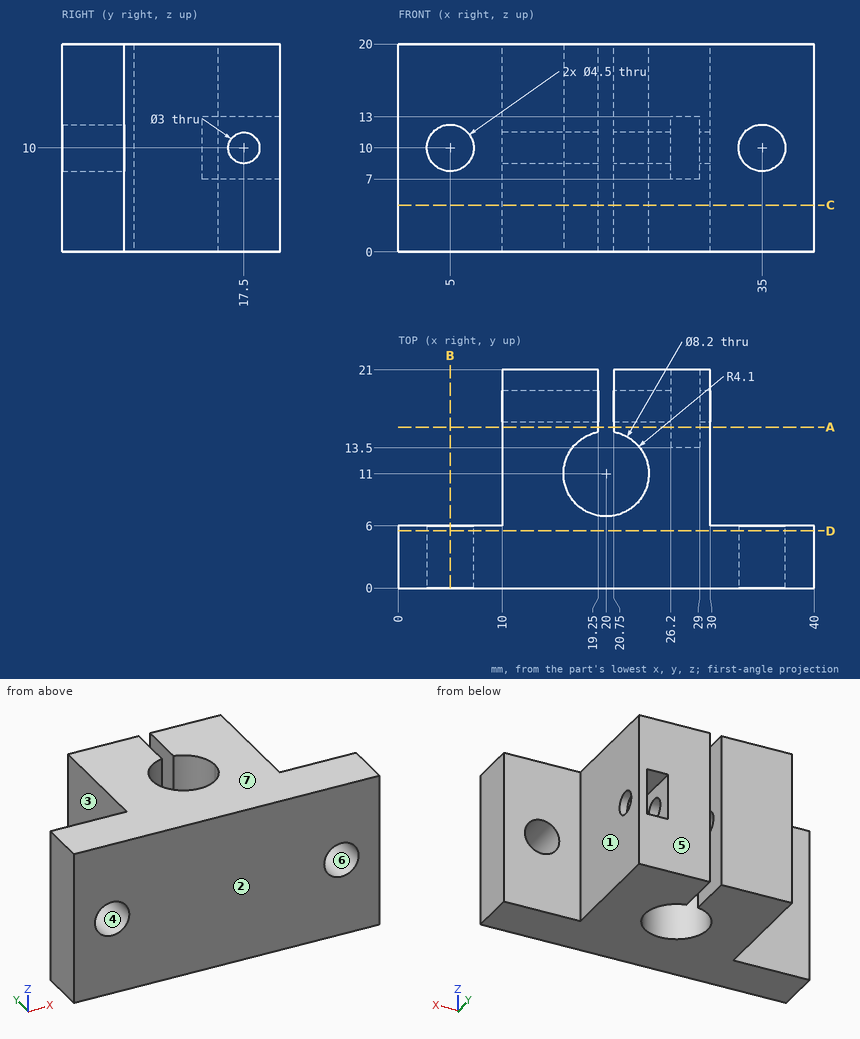
Can you work these out from the drawing? Everything is in mm from the part's minimum corner. A direction names the side the tool comes from. Round coordinates to 2 decimals unless told otherwise and drop trailing zeros. Write each loop counter-clockwise with the first axis right and the second up, starting at its lowest first coordinate (ties: lowest second). Pieces come first, ordered by that corner, then holes. Notation, with made-up numbers: (73.5, 60) - (129.5, 60) arc R20 ccw to (129.5, 93) - close; hole circle Ø6 at (8, 71). An arc over 180 degrees is marked (long way). Use a Markdown table: item, result.
Q1. Please list where these lines run through material, in increasing order: L1, parallel to X at y = 18, z = 12.25; L2, parallel to X at y = 16.5, z = 15; L3, parallel to Z at x = 35, y = 1.25.
Output values:
| item | result |
|---|---|
| L1 | 10 to 19.25, 20.75 to 26.2, 29 to 30 |
| L2 | 10 to 19.25, 20.75 to 30 |
| L3 | 0 to 7.75, 12.25 to 20 |
Q2. For pin 1 (7.5 mm diameter, centred on y = 10.5, z = 9.5, fed in from -X); pin 2 (7 mm diameter, centred on x = 35, z = 10, fed in from +Y); pin 3 (6 mm diameter, centred on x = 35.5, y = 14.5, fed in from -Z); pin 4 (5 mm diameter, centred on y = 16, z = 9.5, fed in from +X), each with a flat end and sliding along its axis, tell me the tip position at first contact or that it passes through.
Output values:
| item | result |
|---|---|
| pin 1 | x = 10 |
| pin 2 | y = 6 |
| pin 3 | through |
| pin 4 | x = 30 |
Q3. Thinking about a two-plate mould opening in Z: for the marked faces 4, 5, 6 and 7, which applies, released by +Z, released by -Z, zero draft, split by the parting line, or undercut?
Output values:
| item | result |
|---|---|
| face 4 | undercut |
| face 5 | zero draft |
| face 6 | undercut |
| face 7 | released by +Z |
Q4. I want a section at A-A (y = 15.5). List the corners of the cut face in (x, z) for me.
Output values:
| item | result |
|---|---|
| outline | (10, 0) - (19.25, 0) - (19.25, 20) - (10, 20) - close; (20.75, 0) - (30, 0) - (30, 20) - (20.75, 20) - close; hole (26.2, 7) - (29, 7) - (29, 13) - (26.2, 13) - close |
Q5. I want a section at C-C (z = 4.5). List the corners of the cut face in (x, y) for me.
Output values:
| item | result |
|---|---|
| outline | (0, 0) - (40, 0) - (40, 6) - (30, 6) - (30, 21) - (20.75, 21) - (20.75, 15.03) arc R4.1 cw to (24.1, 11) arc R4.1 cw (long way) to (19.25, 15.03) - (19.25, 21) - (10, 21) - (10, 6) - (0, 6) - close |
Q6. For the marked faces 1, 2 and 3, which set-ups out of +Z, -Z, +X, -X, +Y, -Y let a thin tool reach every point of the face, with its end or its side?
Output values:
| item | result |
|---|---|
| face 1 | +Z, -Z, +X, +Y |
| face 2 | +Z, -Z, +X, -X, -Y |
| face 3 | +Z, -Z, -X, +Y |
Q7. I want a section at D-D (y = 5.5). List the corners of the cut face in (x, z) for me, plus the area to 3 significant figures.
Output values:
| item | result |
|---|---|
| outline | (0, 0) - (40, 0) - (40, 20) - (0, 20) - close; hole circle Ø4.5 at (5, 10); hole circle Ø4.5 at (35, 10) |
| area | 768 mm2 |
Q8. I want a section at B-B (x = 5). List the corners of the cut face in (y, z) for me.
Output values:
| item | result |
|---|---|
| outline | (0, 0) - (6, 0) - (6, 7.75) - (0, 7.75) - close; (0, 12.25) - (6, 12.25) - (6, 20) - (0, 20) - close |
